Source: CAD feature listing. Evaluate the final solid. Frame: model axes, mm. A direction names the side the tool comes from. Coordinates: 2 decimals unless noted, no trailing zeros. Write each loop counter-clockwise with the first axis right and the second up, starting at its lowest first coordinate (ties: lowest second). Pieces come first, ordered by that corner, then holes. Notation, with made-up numbers: M 56.5,-23.5 L 104.5,-23.5 A12 ccw 104.5,-10.5 Z; hole C 58.5,-4 d7. An arc over 180 degrees is marked long. One line per item, written item: value. Start each with the question number.
Item 1: Cut plane A-A, the plane x = 0. Output: boundary loops of the cut face in (y, z), then the cut area to 3 significant figures.
Item 2: Set-up query: faces 1 (the cylindrical face through (11.923, -3.755, 4.359)), 2 (the cylindrical face through (9.139, -14.334, 0.403)), 3 (the cylindrical face through (-23.977, -1.055, 5.219)). Return all of +Z, -Z, +X, -X, +Y, -Y with unobstructed straight access to the full face (end or side cutting, diameter ignored); none if empty.
Item 3: Ray query, L1, parallel to Z at x = -29.5, y = -3; L2, parallel to X at y = -5, z = 4.5; L3, parallel to Y at x = 13, z = 3.75. Return the intervals inside material, ascending. Write a range as from..to.
Item 4: Cut plane C-C, the plane z = 5.75. Output: boundary loops of the cut face in (x, y), then the cut area to 3 significant figures.
Item 5: Mould query, pull axis X, two halves, no side actions, for faces 4 (the flat face through (-9, 9, 0.818)), 5 (the flat face through (10, -10, 8)), 6 (the cylindrical face through (-4.88, -37.18, 1.61)). Classes: released by +X, released by -X, zero draft, split by the parting line, or undercut.
Item 6: Pin query (flat end, axial travel): P1, Ø17, axis at x = -3, y = 7, coming from the -Z side; P2, Ø3, axis at y = -13.5, z = 3, coming from the -X side; P3, Ø4, axis at x = -23, z = 6, coming from the -Y side. Return the tip coordinate at first contact, or that it passes through.
Autodesk Inventor part; units mm, degrees
ref_plane "Work Plane1" through (-14, -14, 0.8184) normal (0, 0, 1) x (1, 0, 0)
ref_plane "YZ Plane" through (0, 0, 0) normal (1, 0, 0) x (0, 1, 0)
ref_plane "XZ Plane" through (0, 0, 0) normal (0, 1, 0) x (-1, 0, 0)
sketch "Sketch1" plane through (0, 0, 0) normal (0, 0, 1) x (1, 0, 0)
  circle A0 centre (0, 0) radius 37.5
  circle A1 centre (0, 0) radius 12.5
  circle A2 centre (0, 0) radius 26.5 construction
  line L0 (0, 0) -> (0, 26.5) construction
  line L1 (0, 0) -> (10.1411, 24.4828) construction
  circle A3 centre (0, 0) radius 24
  circle A4 centre (0, 0) radius 17
  dimension "d0" = 75
  dimension "d1" = 25
  dimension "d2" = 53
  dimension "d3" = 22.5
  dimension "d19" = 48
  dimension "d22" = 34
extrude "Extrusion1" add sketch "Sketch1" along normal blind 3 contours A0 | A3 | A4
extrude "Extrusion2" add sketch "Sketch1" along normal blind 8 contours A3 | A4
chamfer "Chamfer1" distance 0.25 angle 45 1 edges at (-37.5, 0, 0)
ref_plane "Work Plane1" through (-14, -14, 0.8184) normal (0, 0, 1) x (1, 0, 0)
extrude "Extrusion3" cut sketch "Sketch1" along normal up to surface (0.8184 mm away) contours A4
thread "Thread1"
chamfer "Chamfer2" distance 0.5 angle 45 1 edges at (-24, 0, 8)
hole "Hole2" at (0, 26.5, 0) direction (0, 0, 1) diameter 3 end through all
pattern_circular "Circular Pattern2" count 8 over 360 about axis through (0, 0, -10) along (0, 0, 1) of "Hole2"
properties part number "PWTR-0060" material "Aluminum 6061"
From the geometry:
1. outline: M -37.5,0.25 L -37.25,0 L -28,0 L -28,3 L -37.5,3 Z; M -25,0 L -17,0 L -17,0.82 L -12.5,0.82 L -12.5,8 L -23.5,8 L -24,7.5 L -24,3 L -25,3 Z; M 12.5,0.82 L 17,0.82 L 17,0 L 25,0 L 25,3 L 24,3 L 24,7.5 L 23.5,8 L 12.5,8 Z; M 28,0 L 37.25,0 L 37.5,0.25 L 37.5,3 L 28,3 Z
1. area: 239 mm²
2. face 1: +Z, -Z
2. face 2: -Z
2. face 3: +Z
3. L1: z = 0..3
3. L2: x = -23.47..-11.46, 11.46..23.47
3. L3: y = -20.17..20.17
4. outline: C 0,0 d48; hole C 0,0 d25
4. area: 1,320 mm²
5. face 4: undercut
5. face 5: zero draft
5. face 6: split by the parting line
6. P1: stops at z = 0.82
6. P2: stops at x = -35.53
6. P3: stops at y = -11.62
